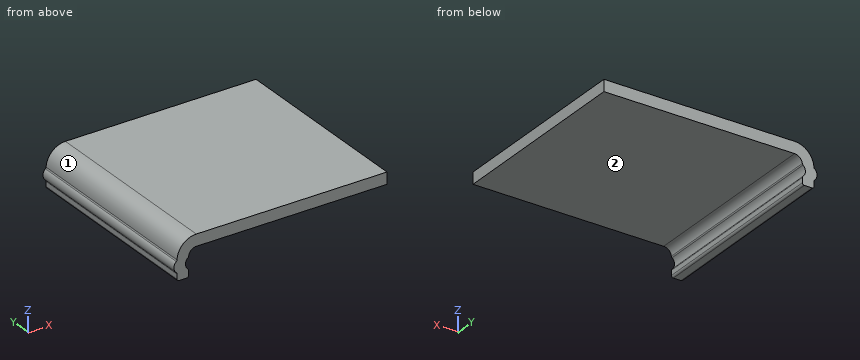
from build123d import *

# Parameters (mm, degrees)
F1_DEPTH = 25
F2_R     = 0.25


with BuildPart() as f1:
    # F0 (on Front) → F1 (new body)
    with BuildSketch(Plane.XZ):
        with BuildLine():
            Line((-24.683436538, 0), (0, 0))
            Line((0, 0), (0, 1.5))
            Line((0, 1.5), (-24.683436538, 1.5))
            ThreePointArc((-24.683436538, 1.5), (-26.451203491, 0.767766953), (-27.183436538, -1))
            ThreePointArc((-27.183436538, -1), (-27.583436538, -1.7483314774), (-27.183436538, -2.4966629547))
            Line((-27.183436538, -2.4966629547), (-27.183436538, -3.4966629547))
            Line((-27.183436538, -3.4966629547), (-25.683436538, -3.4966629547))
            Line((-25.683436538, -3.4966629547), (-25.683436538, -2.4966629547))
            ThreePointArc((-25.683436538, -2.4966629547), (-26.083436538, -1.7483314774), (-25.683436538, -1))
            ThreePointArc((-25.683436538, -1), (-25.3905433192, -0.2928932188), (-24.683436538, 0))
        make_face()
    extrude(amount=F1_DEPTH)

    # F2
    f2_edges = [f1.edges().sort_by_distance(p)[0] for p in [
        (-27.183437, -12.5, -3.496663),
        (-25.683437, -12.5, -3.496663),
        (-25.683437, -12.5, -2.496663),
        (-25.683437, -12.5, -1),
        (-27.183437, -12.5, -2.496663),
        (-27.183437, -12.5, -1),
    ]]
    fillet(f2_edges, radius=F2_R)


solid = f1.part
Could you check a few things on this model? Use its own coordinates, in mm. Face numbers are marked on the shaded views. A direction names the side the tool comes from. Coordinates: 2 decimals unless noted, no trailing zeros. Order: outer loops, then holes, each group sorted by start corner. A loop starts at its lowest first (then second) coordinate and runs counter-clockwise, first axis right, second up.
Q1. Please list where these lines run through material, in increasing order: L1, parallel to Z at x = -19.75, y = -7.5; L2, parallel to X at y = -6.25, z = -3.15; L3, parallel to X at y = -18.5, z = -1.55.
Q2. Suppose I cut it at B-B on z = 0.7. Please give me the cut outline in (x, y).
Q3. Suppose I cut it at A-A on x = -5.25. Please give me the cut outline in (y, z).
Q4. Will this pin go through, and if not, where does the flat tip stop? pin 1 (1 mm diameter, centred on x = -8, z = -1, fed in from +Y).
Q5. Which directions (+Z, -Z, +X, -X, +Y, -Y) give clear straight access to the entire face, cutting with the end or side of a thin tool? Please do the marked faces 1 and 2.
Answer:
1. L1: z = 0 to 1.5
1. L2: x = -27.18 to -25.68
1. L3: x = -27.56 to -26.06
2. outline: (-26.52, -25) - (0, -25) - (0, 0) - (-26.52, 0) - close
3. outline: (-25, 0) - (0, 0) - (0, 1.5) - (-25, 1.5) - close
4. pin 1: passes through
5. face 1: +Z, -X, +Y, -Y
5. face 2: -Z, +X, +Y, -Y
